from build123d import *

# Parameters (mm, degrees)
SKETCH_1_W          = 105
SKETCH_1_H          = 271
EXTRUDE_1_DEPTH     = 2.5
SKETCH_2_R          = 1.6
CUT_EXTRUDE_1_DEPTH = 10
CHAMFER_4_SIZE      = 1
SKETCH_3_W          = 45
SKETCH_3_H          = 34.55
CUT_EXTRUDE_2_DEPTH = 10
SKETCH_4_R          = 2
CUT_EXTRUDE_3_DEPTH = 10
SKETCH_5_R          = 1.6
CUT_EXTRUDE_4_DEPTH = 10
SKETCH_6_R          = 1.6
CUT_EXTRUDE_5_DEPTH = 10
SKETCH_7_R          = 1.65
CUT_EXTRUDE_6_DEPTH = 2
CUT_EXTRUDE_7_REACH = 4.5
SKETCH_8_R          = 1.55
CHAMFER_6_SIZE      = 1.2
SKETCH_9_W          = 30
SKETCH_9_H          = 10
SKETCH_9_H_2        = 20
CUT_EXTRUDE_8_DEPTH = 12
FILLET_1_R          = 2.5


with BuildPart() as part:
    # 草图1 → 凸台-拉伸1 (new body)
    with BuildSketch(Plane(origin=(0, 0, 0), x_dir=(1, 0, 0), z_dir=(0, 1, 0))):
        Rectangle(SKETCH_1_W, SKETCH_1_H)
    extrude(amount=EXTRUDE_1_DEPTH)

    # 草图2 → 切除-拉伸1 (cut)
    with BuildSketch(Plane(origin=(0, 2.5, 0), x_dir=(1, 0, 0), z_dir=(0, 1, 0))):
        with Locations((13.000000181, -3.95)):
            Circle(SKETCH_2_R)
        with Locations((35, -3.95)):
            Circle(SKETCH_2_R)
        with Locations((35, -78.95)):
            Circle(SKETCH_2_R)
        with Locations((13.000000181, -78.95)):
            Circle(SKETCH_2_R)
    extrude(amount=-CUT_EXTRUDE_1_DEPTH, mode=Mode.SUBTRACT)

    # 倒角4
    chamfer_4_edges = [part.edges().sort_by_distance(p)[0] for p in [
        (-52.5, 0, 0),
        (52.5, 0, 0),
    ]]
    chamfer(chamfer_4_edges, length=CHAMFER_4_SIZE)

    # 草图3 → 切除-拉伸2 (cut)
    with BuildSketch(Plane.XZ):
        with Locations((0, 118.225)):
            Rectangle(SKETCH_3_W, SKETCH_3_H)
        with Locations((0, -118.225)):
            Rectangle(SKETCH_3_W, SKETCH_3_H)
    extrude(amount=-CUT_EXTRUDE_2_DEPTH, mode=Mode.SUBTRACT)

    # 草图4 → 切除-拉伸3 (cut)
    with BuildSketch(Plane.XZ):
        with Locations((20.5, -100.95)):
            Circle(SKETCH_4_R)
        with Locations((-20.5, -100.95)):
            Circle(SKETCH_4_R)
        with Locations((-20.5, 100.95)):
            Circle(SKETCH_4_R)
        with Locations((20.5, 100.95)):
            Circle(SKETCH_4_R)
    extrude(amount=-CUT_EXTRUDE_3_DEPTH, mode=Mode.SUBTRACT)

    # 草图5 → 切除-拉伸4 (cut)
    with BuildSketch(Plane(origin=(0, 2.5, 0), x_dir=(1, 0, 0), z_dir=(0, 1, 0))):
        with Locations((-40, 103.95)):
            Circle(SKETCH_5_R)
        with Locations((-30, 103.95)):
            Circle(SKETCH_5_R)
        with Locations((-40, 132.5)):
            Circle(SKETCH_5_R)
        with Locations((-30, 132.5)):
            Circle(SKETCH_5_R)
        with Locations((30, 132.5)):
            Circle(SKETCH_5_R)
        with Locations((40, 132.5)):
            Circle(SKETCH_5_R)
        with Locations((30, 103.95)):
            Circle(SKETCH_5_R)
        with Locations((40, 103.95)):
            Circle(SKETCH_5_R)
        with Locations((40, -103.95)):
            Circle(SKETCH_5_R)
        with Locations((30, -103.95)):
            Circle(SKETCH_5_R)
        with Locations((40, -132.5)):
            Circle(SKETCH_5_R)
        with Locations((30, -132.5)):
            Circle(SKETCH_5_R)
        with Locations((-30, -132.5)):
            Circle(SKETCH_5_R)
        with Locations((-40, -132.5)):
            Circle(SKETCH_5_R)
        with Locations((-30, -103.95)):
            Circle(SKETCH_5_R)
        with Locations((-40, -103.95)):
            Circle(SKETCH_5_R)
    extrude(amount=-CUT_EXTRUDE_4_DEPTH, mode=Mode.SUBTRACT)

    # 草图6 → 切除-拉伸5 (cut)
    with BuildSketch(Plane(origin=(0, 2.5, 0), x_dir=(1, 0, 0), z_dir=(0, 1, 0))):
        with Locations((40, 60)):
            Circle(SKETCH_6_R)
        with Locations((30, 60)):
            Circle(SKETCH_6_R)
        with Locations((40, 40)):
            Circle(SKETCH_6_R)
        with Locations((30, 40)):
            Circle(SKETCH_6_R)
        with Locations((-30, 40)):
            Circle(SKETCH_6_R)
        with Locations((-40, 40)):
            Circle(SKETCH_6_R)
        with Locations((-30, 60)):
            Circle(SKETCH_6_R)
        with Locations((-40, 60)):
            Circle(SKETCH_6_R)
        with Locations((-30, -84.45)):
            Circle(SKETCH_6_R)
        with Locations((-40, -84.45)):
            Circle(SKETCH_6_R)
        with Locations((-30, 13.05)):
            Circle(SKETCH_6_R)
        with Locations((-40, 13.05)):
            Circle(SKETCH_6_R)
    extrude(amount=-CUT_EXTRUDE_5_DEPTH, mode=Mode.SUBTRACT)

    # 草图7 → 切除-拉伸6 (cut)
    with BuildSketch(Plane(origin=(0, 2.5, 0), x_dir=(1, 0, 0), z_dir=(0, 1, 0))):
        with Locations((-22.5, 0)):
            Circle(SKETCH_7_R)
        with Locations((-22.5, -40)):
            Circle(SKETCH_7_R)
        with Locations((-22.5, -80)):
            Circle(SKETCH_7_R)
        with Locations((22.5, -80)):
            Circle(SKETCH_7_R)
        with Locations((22.5, -40)):
            Circle(SKETCH_7_R)
        with Locations((22.5, 0)):
            Circle(SKETCH_7_R)
        with Locations((22.5, 40)):
            Circle(SKETCH_7_R)
        with Locations((22.5, 80)):
            Circle(SKETCH_7_R)
        with Locations((-22.5, 80)):
            Circle(SKETCH_7_R)
        with Locations((-22.5, 40)):
            Circle(SKETCH_7_R)
    extrude(amount=-CUT_EXTRUDE_6_DEPTH, mode=Mode.SUBTRACT)

    # 草图8 → 切除-拉伸7 (cut, up to next)
    with BuildSketch(Plane(origin=(0, 2.5, 0), x_dir=(1, 0, 0), z_dir=(0, 1, 0)), mode=Mode.PRIVATE) as cut_extrude_7_sk1:
        with Locations((-22.5, 80)):
            Circle(SKETCH_8_R)
    cut_extrude_7_tool1 = extrude(cut_extrude_7_sk1.sketch, amount=-CUT_EXTRUDE_7_REACH, mode=Mode.PRIVATE) & part.part
    add(cut_extrude_7_tool1.solids().sort_by_distance((-22.5, 2.5, -80))[0], mode=Mode.SUBTRACT)
    # 草图8 → 切除-拉伸7 (cut, up to next)
    with BuildSketch(Plane(origin=(0, 2.5, 0), x_dir=(1, 0, 0), z_dir=(0, 1, 0)), mode=Mode.PRIVATE) as cut_extrude_7_sk2:
        with Locations((-22.5, 40)):
            Circle(SKETCH_8_R)
    cut_extrude_7_tool2 = extrude(cut_extrude_7_sk2.sketch, amount=-CUT_EXTRUDE_7_REACH, mode=Mode.PRIVATE) & part.part
    add(cut_extrude_7_tool2.solids().sort_by_distance((-22.5, 2.5, -40))[0], mode=Mode.SUBTRACT)
    # 草图8 → 切除-拉伸7 (cut, up to next)
    with BuildSketch(Plane(origin=(0, 2.5, 0), x_dir=(1, 0, 0), z_dir=(0, 1, 0)), mode=Mode.PRIVATE) as cut_extrude_7_sk3:
        with Locations((-22.5, 0)):
            Circle(SKETCH_8_R)
    cut_extrude_7_tool3 = extrude(cut_extrude_7_sk3.sketch, amount=-CUT_EXTRUDE_7_REACH, mode=Mode.PRIVATE) & part.part
    add(cut_extrude_7_tool3.solids().sort_by_distance((-22.5, 2.5, 0))[0], mode=Mode.SUBTRACT)
    # 草图8 → 切除-拉伸7 (cut, up to next)
    with BuildSketch(Plane(origin=(0, 2.5, 0), x_dir=(1, 0, 0), z_dir=(0, 1, 0)), mode=Mode.PRIVATE) as cut_extrude_7_sk4:
        with Locations((-22.5, -40)):
            Circle(SKETCH_8_R)
    cut_extrude_7_tool4 = extrude(cut_extrude_7_sk4.sketch, amount=-CUT_EXTRUDE_7_REACH, mode=Mode.PRIVATE) & part.part
    add(cut_extrude_7_tool4.solids().sort_by_distance((-22.5, 2.5, 40))[0], mode=Mode.SUBTRACT)
    # 草图8 → 切除-拉伸7 (cut, up to next)
    with BuildSketch(Plane(origin=(0, 2.5, 0), x_dir=(1, 0, 0), z_dir=(0, 1, 0)), mode=Mode.PRIVATE) as cut_extrude_7_sk5:
        with Locations((-22.5, -80)):
            Circle(SKETCH_8_R)
    cut_extrude_7_tool5 = extrude(cut_extrude_7_sk5.sketch, amount=-CUT_EXTRUDE_7_REACH, mode=Mode.PRIVATE) & part.part
    add(cut_extrude_7_tool5.solids().sort_by_distance((-22.5, 2.5, 80))[0], mode=Mode.SUBTRACT)
    # 草图8 → 切除-拉伸7 (cut, up to next)
    with BuildSketch(Plane(origin=(0, 2.5, 0), x_dir=(1, 0, 0), z_dir=(0, 1, 0)), mode=Mode.PRIVATE) as cut_extrude_7_sk6:
        with Locations((22.5, -80)):
            Circle(SKETCH_8_R)
    cut_extrude_7_tool6 = extrude(cut_extrude_7_sk6.sketch, amount=-CUT_EXTRUDE_7_REACH, mode=Mode.PRIVATE) & part.part
    add(cut_extrude_7_tool6.solids().sort_by_distance((22.5, 2.5, 80))[0], mode=Mode.SUBTRACT)
    # 草图8 → 切除-拉伸7 (cut, up to next)
    with BuildSketch(Plane(origin=(0, 2.5, 0), x_dir=(1, 0, 0), z_dir=(0, 1, 0)), mode=Mode.PRIVATE) as cut_extrude_7_sk7:
        with Locations((22.5, -40)):
            Circle(SKETCH_8_R)
    cut_extrude_7_tool7 = extrude(cut_extrude_7_sk7.sketch, amount=-CUT_EXTRUDE_7_REACH, mode=Mode.PRIVATE) & part.part
    add(cut_extrude_7_tool7.solids().sort_by_distance((22.5, 2.5, 40))[0], mode=Mode.SUBTRACT)
    # 草图8 → 切除-拉伸7 (cut, up to next)
    with BuildSketch(Plane(origin=(0, 2.5, 0), x_dir=(1, 0, 0), z_dir=(0, 1, 0)), mode=Mode.PRIVATE) as cut_extrude_7_sk8:
        with Locations((22.5, 0)):
            Circle(SKETCH_8_R)
    cut_extrude_7_tool8 = extrude(cut_extrude_7_sk8.sketch, amount=-CUT_EXTRUDE_7_REACH, mode=Mode.PRIVATE) & part.part
    add(cut_extrude_7_tool8.solids().sort_by_distance((22.5, 2.5, 0))[0], mode=Mode.SUBTRACT)
    # 草图8 → 切除-拉伸7 (cut, up to next)
    with BuildSketch(Plane(origin=(0, 2.5, 0), x_dir=(1, 0, 0), z_dir=(0, 1, 0)), mode=Mode.PRIVATE) as cut_extrude_7_sk9:
        with Locations((22.5, 40)):
            Circle(SKETCH_8_R)
    cut_extrude_7_tool9 = extrude(cut_extrude_7_sk9.sketch, amount=-CUT_EXTRUDE_7_REACH, mode=Mode.PRIVATE) & part.part
    add(cut_extrude_7_tool9.solids().sort_by_distance((22.5, 2.5, -40))[0], mode=Mode.SUBTRACT)
    # 草图8 → 切除-拉伸7 (cut, up to next)
    with BuildSketch(Plane(origin=(0, 2.5, 0), x_dir=(1, 0, 0), z_dir=(0, 1, 0)), mode=Mode.PRIVATE) as cut_extrude_7_sk10:
        with Locations((22.5, 80)):
            Circle(SKETCH_8_R)
    cut_extrude_7_tool10 = extrude(cut_extrude_7_sk10.sketch, amount=-CUT_EXTRUDE_7_REACH, mode=Mode.PRIVATE) & part.part
    add(cut_extrude_7_tool10.solids().sort_by_distance((22.5, 2.5, -80))[0], mode=Mode.SUBTRACT)

    # 倒角6
    chamfer_6_edges = [part.edges().sort_by_distance(p)[0] for p in [
        (11.400000181, 0, 3.95),
        (-41.6, 0, -40),
        (33.4, 0, 78.95),
        (-31.6, 0, -60),
        (-41.6, 0, -60),
        (-31.6, 0, 84.45),
        (28.4, 0, -60),
        (38.4, 0, -40),
        (28.4, 0, -40),
        (-31.6, 0, -40),
        (-41.6, 0, -13.05),
        (-31.6, 0, -13.05),
        (-41.6, 0, 84.45),
        (11.400000181, 0, 78.95),
        (38.4, 0, -60),
        (33.4, 0, 3.95),
    ]]
    chamfer(chamfer_6_edges, length=CHAMFER_6_SIZE)

    # 草图9 → 切除-拉伸8 (cut)
    with BuildSketch(Plane.XZ):
        with Locations((0, -11.05)):
            Rectangle(SKETCH_9_W, SKETCH_9_H)
        with Locations((0, -36.05)):
            Rectangle(SKETCH_9_W, SKETCH_9_H_2)
    extrude(amount=-CUT_EXTRUDE_8_DEPTH, mode=Mode.SUBTRACT)

    # 圆角1
    fillet_1_edges = [part.edges().sort_by_distance(p)[0] for p in [
        (15, 1.25, -6.05),
        (15, 1.25, -16.05),
        (-15, 1.25, -16.05),
        (-15, 1.25, -6.05),
        (15, 1.25, -46.05),
        (-15, 1.25, -46.05),
        (-15, 1.25, -26.05),
        (15, 1.25, -26.05),
    ]]
    fillet(fillet_1_edges, radius=FILLET_1_R)


solid = part.part
Geometry: final body of the model. Coordinates: model frame, mm. Coordinates: 2 decimals unless noted, no trailing zeros.
(1) Section query A-A (y = 1.8). State how many separate pieces and enclosed holes the cut face has, plus the area to 3 significant figures.
(2) First-contact query: pin 1 (1.2 mm diameter, centred on x = -5, y = 1.5, fed in from -Z); pin 2 (1 mm diameter, centred on x = 23, z = -1, fed in from +Y). Flat tips, straight axial feed; report the tip coordinate or a pass-through.
(3) Material intervals for probe 1 along X at (y, z) = (1.65, -60); probe 2 along X at (y, z) = (1.25, 0); probe 3 along X at (y, z) = (1.85, -12), sorted ascending.
Solution:
1. separate pieces: 1
1. enclosed holes: 44
1. area: 24,100 mm2
2. pin 1: stops at z = -100.95
2. pin 2: stops at y = 0.5
3. probe 1: x = -52.5 to -41.6, -38.4 to -31.6, -28.4 to 28.4, 31.6 to 38.4, 41.6 to 52.5
3. probe 2: x = -52.5 to -24.15, -20.85 to 20.85, 24.15 to 52.5
3. probe 3: x = -52.5 to -41.21, -38.79 to -31.21, -28.79 to -15, 15 to 52.5
